```python
from build123d import *

# Parameters (mm, degrees)
CYLINDER_R      = 2
CYLINDER_DEPTH  = 102
SPHERE_ANGLE    = 180
SPHERE001_ANGLE = 180


with BuildPart() as cylinder:
    # Cylinder → Cylinder (new body)
    with BuildSketch(Plane(origin=(-1, 50, 3.4), x_dir=(0, 0, 1), z_dir=(1, 0, 0))):
        Circle(CYLINDER_R)
    extrude(amount=CYLINDER_DEPTH)


with BuildPart() as sphere:
    # Sphere → Sphere (revolve)
    with BuildSketch(Plane(origin=(0, 50, 3.5), x_dir=(0, 1, 0), z_dir=(1, 0, 0))):
        with BuildLine():
            ThreePointArc((0, -4), (4, 0), (0, 4))
            Line((0, 4), (0, -4))
        make_face()
    revolve(axis=Axis((0, 50, 3.5), (0, 0, 1)), revolution_arc=SPHERE_ANGLE)


with BuildPart() as fusion:
    # Sphere001 → Sphere001 (revolve)
    with BuildSketch(Plane(origin=(100, 50, 3.5), x_dir=(0, -1, 0), z_dir=(-1, 0, 0))):
        with BuildLine():
            ThreePointArc((0, -4), (4, 0), (0, 4))
            Line((0, 4), (0, -4))
        make_face()
    revolve(axis=Axis((100, 50, 3.5), (0, 0, 1)), revolution_arc=SPHERE001_ANGLE)

    # Fusion: union Cylinder, Sphere
    add(cylinder.part)
    add(sphere.part)


with BuildPart() as fusion_1:
    # Fusion placement: moved
    add(fusion.part.moved(Location((0, -50, 0))))


solid = fusion_1.part
```
Read the model definition and answer for the solid it produces. Units are mm, in the model's axes. Give positions to 0.01 mm unless a question says otherwise; leave off trailing zeros. Write each loop counter-clockwise with the first axis right and the second up, starting at its lowest first coordinate (ties: lowest second). Pieces come first, ordered by that corner, then holes. Notation, with made-up numbers: (-12.75, 35.25) -> (-3.75, 35.25) arc R18 ccw to (-3.75, 41.25) -> close; hole circle Ø4 at (81.25, -10.75). An arc over 180 degrees is marked (long way). Answer in a Markdown table with one row per item.
1) Section A-A on y = 0 is taken. Give the vertices of the cut face in (x, z), plus the area to 3 significant figures.
Results list:
| item | result |
|---|---|
| outline | (0, -0.5) -> (0, 1.4) -> (100, 1.4) -> (100, -0.5) arc R4 ccw to (100, 7.5) -> (100, 5.4) -> (0, 5.4) -> (0, 7.5) arc R4 ccw to start |
| area | 450 mm^2 |
2) Straight lines are drawn through the part: line 1 (X direction, y = 1.5, z = 6.25); line 2 (X direction, y = 2, z = 5.75); line 3 (Y direction, x = 42, z = 3.5). For each, find the intervals that lie inside material, in ascending order. Write a range as [from, to].
Results list:
| item | result |
|---|---|
| line 1 | [-2.49, 0], [100, 102.49] |
| line 2 | [-2.63, 0], [100, 102.63] |
| line 3 | [-2, 2] |
3) Section B-B on z = 4 is taken. Give the vertices of the cut face in (x, y).
Results list:
| item | result |
|---|---|
| outline | (0, -3.97) -> (0, -1.91) -> (100, -1.91) -> (100, -3.97) arc R3.97 ccw to (100, 3.97) -> (100, 1.91) -> (0, 1.91) -> (0, 3.97) arc R3.97 ccw to start |
4) Section C-C on x = 22 is taken. Give the vertices of the cut face in (y, z).
Results list:
| item | result |
|---|---|
| outline | circle Ø4 at (0, 3.4) |
5) Each of these flat-tipped pins is pushed along its axis until it touches: pin 1 Ø1 at (y, z) = (-2.5, 5) entering from +X; pin 2 Ø1.5 at (y, z) = (-3, 5) entering from -X; pin 3 Ø1 at (x, z) = (21.5, 0.5) entering from +Y; pin 4 Ø4 at (x, y) = (89.5, -1) entering from -Z. Where does it stop, or does it pass through?
Results list:
| item | result |
|---|---|
| pin 1 | x = 103.19 |
| pin 2 | x = -3.04 |
| pin 3 | through |
| pin 4 | z = 1.4 |
